The model under review builds one solid part; all positions refer to its coordinate system, in mm. A direction names the side the tool comes from. Round coordinates to 2 decimals unless told otherwise and drop trailing zeros. Write each loop counter-clockwise with the first axis right and the second up, starting at its lowest first coordinate (ties: lowest second). Pieces come first, ordered by that corner, then holes. Notation, with made-up numbers: (21, -29.75) - (36, -29.75) arc R19 ccw to (36, -7.75) - close; hole circle Ø11 at (75.5, 32.25). An arc over 180 degrees is marked (long way). Write each question's results on one line, items separated by ' | '.
Autodesk Inventor part; units mm, degrees
ref_plane "YZ Plane" through (0, 0, 0) normal (1, 0, 0) x (0, 1, 0)
ref_plane "XZ Plane" through (0, 0, 0) normal (0, 1, 0) x (-1, 0, 0)
ref_plane "XY Plane" through (0, 0, 0) normal (0, 0, 1) x (1, 0, 0)
sketch "Sketch1" plane through (0, 0, 0) normal (0, 0, 1) x (1, 0, 0)
  circle A0 centre (2.8434, 6.5346) radius 4.064 construction
  circle A1 centre (-76.1973, 37.0416) radius 3.9624 construction
  arc A2 (-75.0852, 40.0155) -> (-77.3716, 34.0917) centre (-76.1973, 37.0416) ccw
  line L0 (-75.0852, 40.0155) -> (4.2669, 10.3412)
  line L1 (1.3404, 2.7588) -> (-77.3716, 34.0917)
  arc A3 (1.3404, 2.7588) -> (4.2669, 10.3412) centre (2.8434, 6.5346) ccw
  line L2 (4.6172, 11.2778) -> (-74.7349, 40.9521)
  arc A4 (-74.7349, 40.9521) -> (-77.7414, 33.1626) centre (-76.1973, 37.0416) ccw
  line L3 (-77.7414, 33.1626) -> (0.9705, 1.8297)
  arc A5 (0.9705, 1.8297) -> (4.6172, 11.2778) centre (2.8434, 6.5346) ccw
  point P0 (0, 0)
  dimension "d0" = 6.35
  dimension "d1" = 1
extrude "Extrusion1" add sketch "Sketch1" against normal blind 5
properties part number "Single Indexer tensioner band"
Q1. For probe 1 along Y at (x, z) = (-52, -0.35); probe 2 along Y at (x, z) = (-70, -1.65), list the stretches that pass through material, from the lowest coordinate up.
Evaluation:
probe 1: y = 22.92 to 23.99, 31.38 to 32.45 | probe 2: y = 30.08 to 31.16, 38.11 to 39.18
Q2. The part is to be moulded in two halves that separate along X. For faces 1 (the cylindrical face through (-80.06, 38.63, -2.46)), 2 (the flat face through (-38.9, 17.7, -2.5)), 3 (the cylindrical face through (-79.134, 38.249, -2.465)), say which applies: released by +X, released by -X, zero draft, split by the parting line, or undercut.
Evaluation:
face 1: split by the parting line | face 2: released by -X | face 3: undercut
Q3. We need section C-C (x = -13.5). State the section outline as (y, z) points, plus the area to 3 significant figures.
Evaluation:
outline: (7.59, -5) - (8.67, -5) - (8.67, 0) - (7.59, 0) - close; (16.99, -5) - (18.05, -5) - (18.05, 0) - (16.99, 0) - close | area: 10.7 mm^2
Q4. Tool access review of faces 4 (the flat face through (-36, 25.4, -2.5)), 5 (the flat face through (-36, 26, -5)): name each direction out of +Z, -Z, +X, -X, +Y, -Y from which nothing blocks a thin tool from reaching the whole face with its end or side.
Evaluation:
face 4: +Z, -Z | face 5: -Z, +X, -X, +Y, -Y
Q5. We need section B-B (y = 4.5). State the section outline as (x, z) points, plus the area to 3 significant figures.
Evaluation:
outline: (-5.74, -5) - (-3.03, -5) - (-3.03, 0) - (-5.74, 0) - close; (6.36, -5) - (7.48, -5) - (7.48, 0) - (6.36, 0) - close | area: 19.1 mm^2
Q6. Insertion check: P1, Ø1.5, axis at x = -58, z = -2, coming from the -Y side; P2, Ø2, axis at x = -49.5, z = -2, coming from the +Y side. Each pin has a flat end and moves straight along its axis. Give the tip position at first contact, or say it passes through.
Evaluation:
P1: stops at y = 25.01 | P2: stops at y = 31.89
Q7. We need section A-A (z = -2.5). State the section outline as (x, y) points, plus the area to 3 significant figures.
Evaluation:
outline: (-77.74, 33.16) - (0.97, 1.83) arc R5.06 ccw (long way) to (4.62, 11.28) - (-74.73, 40.95) arc R4.18 ccw to start; hole (-77.37, 34.09) - (1.34, 2.76) arc R4.06 ccw (long way) to (4.27, 10.34) - (-75.09, 40.02) arc R3.18 ccw to start | area: 195 mm^2
